The model under review builds one solid part; all positions refer to its coordinate system, in mm. Give positions to 0.01 mm unless a question says otherwise; leave off trailing zeros. Loops run counter-clockwise (first coordinate to the right, second up) from the corner with the lowest first, then second, coordinate; pieces in that order, holes last. Notation, with made-up numbers: M 17,63 L 28,63 A23 cw 28,102 Z; hole C 45,61.25 d5. An arc over 180 degrees is marked long. Write item = value, one per line. Start each with the question number.
1. We need section B-B on x = -10. Give the boundary of the cut face in (y, z) (3 decimals), then the cut area to 3 significant figures.
2. Wall thickness on line 1 along Z through (x, y) = (239, 14); line 2 along Z through (x, y) = (-11, 14.5); line 3 along Y through (x, z) = (111, 57.5) (3 decimals): over which ranges is each line inside the solid? List them lowest first. Write a range as from..to.
3. We need section C-C on z = 18. Give the boundary of the cut face in (x, y) (3 decimals), then the cut area to 3 significant figures.
4. We need section A-A on y = 11.5. Give the boundary of the cut face in (x, z).
5. Draft analysis for pull direction Z (two halves, no side actions). For faces 1 (the face through (-5, 9, -125)), 2 (the face through (-5, 18, 91)), 3 (the face through (2, 8.475, 49)), 4 (the face through (-5, 9, 125)), state which applies: pulls with the +Z half, pulls with the -Z half, needs draft (parallel to the pull), parting line crosses it, or undercut.
from build123d import *

# Parameters (mm, degrees)
SKETCH1_W           = 735
SKETCH1_H           = 250
BOSS_EXTRUDE1_DEPTH = 18
CUT_EXTRUDE1_DEPTH  = 9.525


with BuildPart() as part:
    # Sketch1 → Boss-Extrude1 (new body)
    with BuildSketch(Plane(origin=(0, 0, 0), x_dir=(1, 0, 0), z_dir=(0, 1, 0))):
        Rectangle(SKETCH1_W, SKETCH1_H)
    extrude(amount=BOSS_EXTRUDE1_DEPTH)

    # Sketch4 → Cut-Extrude1 (cut)
    with BuildSketch(Plane(origin=(0, 18, 0), x_dir=(1, 0, 0), z_dir=(0, 1, 0))):
        Polygon((-390.644484973, -45), (-25.4, -45), (-25.4, -6.9), (25.4, -6.9), (25.4, -45), (418.930169805, -45), (418.930169805, -57.7), (-390.644484973, -57.7), align=None)
    extrude(amount=-CUT_EXTRUDE1_DEPTH, mode=Mode.SUBTRACT)


solid = part.part
Final values:
q1.outline = M 0,-125 L 18,-125 L 18,6.9 L 8.475,6.9 L 8.475,57.7 L 18,57.7 L 18,125 L 0,125 Z
q1.area = 4,020 mm²
q2.line_1 = -125..45, 57.7..125
q2.line_2 = -125..6.9, 57.7..125
q2.line_3 = 0..8.475
q3.outline = M -367.5,0 L 367.5,0 L 367.5,18 L 25.4,18 L 25.4,8.475 L -25.4,8.475 L -25.4,18 L -367.5,18 Z
q3.area = 12,700 mm²
q4.outline = M -367.5,-125 L 367.5,-125 L 367.5,45 L 25.4,45 L 25.4,6.9 L -25.4,6.9 L -25.4,45 L -367.5,45 Z; M -367.5,57.7 L 367.5,57.7 L 367.5,125 L -367.5,125 Z
q5.face_1 = pulls with the -Z half
q5.face_2 = needs draft
q5.face_3 = undercut
q5.face_4 = pulls with the +Z half
